```python
from build123d import *

# Parameters (mm, degrees)
SKETCH1_R           = 9
SKETCH1_R_2         = 7.75
BOSS_EXTRUDE1_DEPTH = 3
SKETCH2_R           = 9
SKETCH2_R_2         = 5
BOSS_EXTRUDE2_DEPTH = 1
THREAD2_PITCH       = 1
THREAD2_TO          = 4


with BuildPart() as part:
    # Sketch1 → Boss-Extrude1 (new body)
    with BuildSketch(Plane(origin=(0, 0, 0), x_dir=(1, 0, 0), z_dir=(0, 1, 0))):
        with Locations(Location((0, 0, 0), (0, 0, 270))):
            Circle(SKETCH1_R)
        with Locations(Location((0, 0, 0), (0, 0, 270))):
            Circle(SKETCH1_R_2, mode=Mode.SUBTRACT)
    extrude(amount=BOSS_EXTRUDE1_DEPTH)

    # Sketch2 → Boss-Extrude2 (add)
    with BuildSketch(Plane(origin=(0, 3, 0), x_dir=(1, 0, 0), z_dir=(0, 1, 0))):
        with Locations(Location((0, 0, 0), (0, 0, 270))):
            Circle(SKETCH2_R)
        with Locations(Location((0, 0, 0), (0, 0, 270))):
            Circle(SKETCH2_R_2, mode=Mode.SUBTRACT)
    extrude(amount=BOSS_EXTRUDE2_DEPTH)

    # Thread2: arcs per turn and ends read off the stored shape
    # Thread2: the profile of Thread Profile2 profile screwed along a right-hand helix through 4 turns, 8 arcs to a turn; built about Z, then put on its axis
    thread2_z = Axis((0, 0, 0), (0, 0, 1))
    thread2_corners = [(7.7497, 0, -0.000173205), (8.291265875, 0, 0.312499999), (8.291265875, 0, 0.437499999), (7.7497, 0, 0.750173202)]
    with BuildLine(mode=Mode.PRIVATE) as thread2_profile:
        Line(thread2_corners[0], thread2_corners[1])
        Line(thread2_corners[1], thread2_corners[2])
        Line(thread2_corners[2], thread2_corners[3])
        Line(thread2_corners[3], thread2_corners[0])
    thread2_cap = Face(thread2_profile.wire())
    thread2_turn_angles = [0, 22.5, 45, 67.5, 90, 112.5, 135, 157.5, 180, 202.5, 225, 247.5, 270, 292.5, 315, 337.5, 360]
    thread2_turn_weights = [1, 0.9238795325112867, 1, 0.9238795325112867, 1, 0.9238795325112867, 1, 0.9238795325112867, 1, 0.9238795325112867, 1, 0.9238795325112867, 1, 0.9238795325112867, 1, 0.9238795325112867, 1]
    thread2_turn_rails = [Edge.make_bspline([Vector(p[0], p[1], 0).rotate(thread2_z, thread2_turn_angles[k]) / thread2_turn_weights[k] + Vector(0, 0, p[2] + THREAD2_PITCH * thread2_turn_angles[k] / 360) for k in range(17)], [0, 0, 0, 1, 1, 2, 2, 3, 3, 4, 4, 5, 5, 6, 6, 7, 7, 8, 8, 8], 2, thread2_turn_weights) for p in thread2_corners]
    thread2_turn_sides = [Face.make_surface_from_curves(thread2_turn_rails[p[0]], thread2_turn_rails[p[1]]) for p in [(0, 1), (1, 2), (2, 3), (3, 0)]]
    thread2 = Plane(origin=(0, -1, 0), x_dir=(1, 0, 0), z_dir=(0, 1, 0)) * split(Solid(Shell([*[p.moved(Location((0, 0, THREAD2_PITCH * i))) for i in range(4) for p in thread2_turn_sides], thread2_cap, thread2_cap.rotate(thread2_z, 1440).moved(Location((0, 0, THREAD2_PITCH * 1440 / 360)))])), bisect_by=Plane.XY.offset(THREAD2_TO), keep=Keep.BOTTOM, mode=Mode.PRIVATE)
    add(thread2, mode=Mode.SUBTRACT)


solid = part.part
```
Build history of the part. All positions in model axes, mm. Coordinates: 2 decimals unless noted, no trailing zeros. Order: outer loops, then holes, each group sorted by start corner. A loop starts at its lowest first (then second) coordinate and runs counter-clockwise, first axis right, second up. Notation, with made-up numbers: M 28,80.5 L 64,80.5 A22 cw 64,98.5 Z; hole C 22,2 d1. An arc over 180 degrees is marked long. One line per question, with ' | ' between items. Start each with the question number.
1. Flat gauge pins, fed straight in: P1, Ø1.5, axis at y = 1.5, z = 3.5, coming from the -X side; P2, Ø1, axis at y = 2.5, z = 1.5, coming from the -X side; P3, Ø1, axis at y = 2, z = -4.5, coming from the -X side. Where does each tip first touch, or does it go through?
2. Cut at A-A (y = 3.45). Write the cut outline in (x, z), plus the area to 3 significant figures.
3. Wall check: line 1 along X through (y, z) = (0.9, 0); line 2 along X through (y, z) = (3.5, 0); line 3 along Y through (x, z) = (-7.25, -3). Give the ranges that are in metal, low to high. Write a range as [from, to].
4. Mould opens along Z. For faces 1 (the face through (-4, 4, 4)), 2 (the face through (-4, 3, 4)), 3 (the face through (2.703, 1.972, 8.584)) say: +Z half, -Z half, draft (parallel to the pull), parting line (faces both ways), or undercut.
The answers:
1) P1: stops at x = -8.57 | P2: stops at x = -8.94 | P3: stops at x = -8.06
2) outline: C 0,0 d18; hole C 0,0 d10 | area: 176 mm2
3) line 1: x = [-9, -8.29], [7.75, 9] | line 2: x = [-9, -5], [5, 9] | line 3: y = [0.13, 0.49], [1.13, 1.49], [2.13, 2.49], [3, 4]
4) face 1: draft | face 2: undercut | face 3: parting line
